```python
from build123d import *

# Parameters (mm, degrees)
SKETCH_1_W                = 290
SKETCH_1_H                = 290
EXTRUDE_1_DEPTH           = 4
EXTRUDE_2_DEPTH           = 76
SKETCH_4_W                = 6
SKETCH_4_H                = 290
EXTRUDE_3_DEPTH           = 76
CUT_EXTRUDE_12_DEPTH      = 334.95358959
CUT_EXTRUDE_12_DEPTH_BACK = 334.95358959
SKETCH_17_R               = 19.5
SKETCH_17_R_2             = 3
SKETCH_18_W               = 4
SKETCH_18_H               = 290
EXTRUDE_4_DEPTH           = 70
CUT_EXTRUDE_13_DEPTH      = 334.95358959
CUT_EXTRUDE_13_DEPTH_BACK = 334.95358959
SKETCH_14_W               = 80
SKETCH_14_H               = 30
CUT_EXTRUDE_9_DEPTH       = 20
EXTRUDE_1_2_OUTLINE_W     = 176
EXTRUDE_1_2_OUTLINE_H     = 4
EXTRUDE_1_2_DEPTH         = 20
CUT_EXTRUDE_10_DEPTH      = 334.95358959
CUT_EXTRUDE_10_DEPTH_BACK = 334.95358959
SKETCH_15_R               = 3
SKETCH_15_R_2             = 3.5
SKETCH_7_R                = 1.9
CUT_EXTRUDE_3_DEPTH       = 10
FILLET_1_R                = 2
SKETCH_21_R               = 3.6
SKETCH_21_W               = 19.5
SKETCH_21_H               = 13.5
CUT_EXTRUDE_14_DEPTH      = 10
CHAMFER_1_SIZE            = 2
FILLET_2_R                = 3
CHAMFER_2_SIZE            = 3


# Read off the part's stored shape, not the designer's step: Вытянуть-Тонкостенный1
with BuildPart() as part:
    # Эскиз1 → Extrude 1 (new body)
    with BuildSketch(Plane(origin=(0, 0, 0), x_dir=(1, 0, 0), z_dir=(0, 1, 0))):
        Rectangle(SKETCH_1_W, SKETCH_1_H)
    extrude(amount=EXTRUDE_1_DEPTH)

    # Эскиз2 → Бобышка-Вытянуть2 (add)
    with BuildSketch(Plane(origin=(0, 4, 0), x_dir=(1, 0, 0), z_dir=(0, 1, 0))):
        Polygon((145, 145), (145, 0.239524614), (145, -145), (-139, -145), (-139, -139), (139, -139), (139, 139), (-139, 139), (-139, 145), align=None)
    extrude(amount=EXTRUDE_2_DEPTH)

    # Эскиз4 → Бобышка-Вытянуть3 (add)
    with BuildSketch(Plane(origin=(0, 4, 0), x_dir=(1, 0, 0), z_dir=(0, 1, 0))):
        with Locations((-142, 0)):
            Rectangle(SKETCH_4_W, SKETCH_4_H)
    extrude(amount=EXTRUDE_3_DEPTH)

    # Эскиз17 → Вырез-Вытянуть12 (cut, two sides: drawn at the far end of the back side and taken through both)
    with BuildSketch(Plane.XY.offset(145).offset(-CUT_EXTRUDE_12_DEPTH_BACK)):
        with Locations((81, 33)):
            Circle(SKETCH_17_R)
        with Locations((57.43, 56.57)):
            Circle(SKETCH_17_R_2)
        with Locations((104.57, 56.57)):
            Circle(SKETCH_17_R_2)
        with Locations((104.57, 9.43)):
            Circle(SKETCH_17_R_2)
        with Locations((57.43, 9.43)):
            Circle(SKETCH_17_R_2)
    extrude(amount=CUT_EXTRUDE_12_DEPTH + CUT_EXTRUDE_12_DEPTH_BACK, mode=Mode.SUBTRACT)

    # Эскиз18 → Бобышка-Вытянуть4 (add)
    with BuildSketch(Plane(origin=(0, 4, 0), x_dir=(1, 0, 0), z_dir=(0, 1, 0))):
        with Locations((39, 0)):
            Rectangle(SKETCH_18_W, SKETCH_18_H)
    extrude(amount=EXTRUDE_4_DEPTH)

    # Эскиз19 → Вырез-Вытянуть13 (cut, two sides: drawn at the far end of the back side and taken through both)
    with BuildSketch(Plane(origin=(145, 0, 0), x_dir=(0, 0, -1), z_dir=(1, 0, 0)).offset(-CUT_EXTRUDE_13_DEPTH_BACK)):
        Polygon((-80, 24), (80, 24), (119, 80), (-119, 80), align=None)
    extrude(amount=CUT_EXTRUDE_13_DEPTH + CUT_EXTRUDE_13_DEPTH_BACK, mode=Mode.SUBTRACT)

    # Эскиз14 → Вырез-Вытянуть9 (cut)
    with BuildSketch(Plane(origin=(0, 4, 0), x_dir=(1, 0, 0), z_dir=(0, 1, 0))):
        with Locations((81, 120)):
            Rectangle(SKETCH_14_W, SKETCH_14_H)
        with Locations((81, -120)):
            Rectangle(SKETCH_14_W, SKETCH_14_H)
    extrude(amount=-CUT_EXTRUDE_9_DEPTH, mode=Mode.SUBTRACT)

    # Extrude 1 2 outline → Extrude 1 2 (add)
    with BuildSketch(Plane(origin=(0, 4, 0), x_dir=(1, 0, 0), z_dir=(0, 1, 0))):
        with Locations((-51, 67)):
            Rectangle(EXTRUDE_1_2_OUTLINE_W, EXTRUDE_1_2_OUTLINE_H)
        with Locations((-51, -67)):
            Rectangle(EXTRUDE_1_2_OUTLINE_W, EXTRUDE_1_2_OUTLINE_H)
    extrude(amount=EXTRUDE_1_2_DEPTH)

    # Эскиз15 → Вырез-Вытянуть10 (cut, two sides: drawn at the far end of the back side and taken through both)
    with BuildSketch(Plane.ZY.offset(145).offset(-CUT_EXTRUDE_10_DEPTH_BACK)):
        with Locations((0, 65)):
            Circle(SKETCH_15_R)
        with Locations((125, 65)):
            Circle(SKETCH_15_R_2)
        with Locations((-125, 65)):
            Circle(SKETCH_15_R_2)
        with Locations((-125, 15)):
            Circle(SKETCH_15_R_2)
        with Locations((125, 15)):
            Circle(SKETCH_15_R_2)
        with Locations((0, 15)):
            Circle(SKETCH_15_R)
    extrude(amount=CUT_EXTRUDE_10_DEPTH + CUT_EXTRUDE_10_DEPTH_BACK, mode=Mode.SUBTRACT)

    # Эскиз7 → Вырез-Вытянуть3 (cut)
    with BuildSketch(Plane(origin=(0, 4, 0), x_dir=(1, 0, 0), z_dir=(0, 1, 0))):
        with Locations(Location((-109, 55, 0), (0, 0, 270))):
            Circle(SKETCH_7_R)
        with Locations(Location((1, 55, 0), (0, 0, 90))):
            Circle(SKETCH_7_R)
        with Locations(Location((1, -55, 0), (0, 0, 270))):
            Circle(SKETCH_7_R)
        with Locations(Location((-109, -55, 0), (0, 0, 90))):
            Circle(SKETCH_7_R)
        with Locations(Location((-134, 60, 0), (0, 0, 270))):
            Circle(SKETCH_7_R)
        with Locations(Location((-134, -60, 0), (0, 0, 90))):
            Circle(SKETCH_7_R)
        with Locations(Location((134, 134, 0), (0, 0, 270))):
            Circle(SKETCH_7_R)
        with Locations(Location((134, -134, 0), (0, 0, 90))):
            Circle(SKETCH_7_R)
        with Locations(Location((134, -60, 0), (0, 0, 270))):
            Circle(SKETCH_7_R)
        with Locations(Location((134, 60, 0), (0, 0, 90))):
            Circle(SKETCH_7_R)
        with Locations(Location((46, -60, 0), (0, 0, 90))):
            Circle(SKETCH_7_R)
        with Locations(Location((46, 60, 0), (0, 0, 270))):
            Circle(SKETCH_7_R)
        with Locations(Location((45, 45, 0), (0, 0, 270))):
            Circle(SKETCH_7_R)
        with Locations(Location((135, 45, 0), (0, 0, 270))):
            Circle(SKETCH_7_R)
        with Locations(Location((45, -45, 0), (0, 0, 270))):
            Circle(SKETCH_7_R)
        with Locations(Location((135, -45, 0), (0, 0, 270))):
            Circle(SKETCH_7_R)
        with Locations(Location((-121, 124.5, 0), (0, 0, 270))):
            Circle(SKETCH_7_R)
        with Locations(Location((-121, 74.5, 0), (0, 0, 270))):
            Circle(SKETCH_7_R)
        with Locations(Location((19, 124.5, 0), (0, 0, 270))):
            Circle(SKETCH_7_R)
        with Locations(Location((19, 74.5, 0), (0, 0, 270))):
            Circle(SKETCH_7_R)
        with Locations(Location((19, -74.5, 0), (0, 0, 90))):
            Circle(SKETCH_7_R)
        with Locations(Location((19, -124.5, 0), (0, 0, 90))):
            Circle(SKETCH_7_R)
        with Locations(Location((-121, -74.5, 0), (0, 0, 90))):
            Circle(SKETCH_7_R)
        with Locations(Location((-121, -124.5, 0), (0, 0, 90))):
            Circle(SKETCH_7_R)
    extrude(amount=-CUT_EXTRUDE_3_DEPTH, mode=Mode.SUBTRACT)

    # Скругление1
    fillet_1_edges = [part.edges().sort_by_distance(p)[0] for p in [
        (-142, 24, -80),
        (-142, 24, 80),
        (39, 24, -80),
        (-139, 24, 0),
        (-51, 24, -65),
        (37, 24, 0),
        (-51, 24, 65),
        (142, 24, 80),
        (139, 4, 0),
        (139, 42, 139),
        (139, 42, -139),
        (-51, 4, 139),
        (37, 39, 139),
        (39, 74, 139),
        (41, 39, 139),
        (-139, 42, 139),
        (-139, 4, 104),
        (142, 24, -80),
        (121, 2, 135),
        (41, 2, 135),
        (41, 4, 137),
        (41, 2, 105),
        (41, 4, 0),
        (41, 2, -105),
        (41, 2, -135),
        (41, 4, -137),
        (41, 39, -139),
        (121, 2, 105),
        (121, 2, -105),
        (121, 2, -135),
        (-139, 4, -104),
        (-139, 42, -139),
        (39, 74, -139),
        (37, 39, -139),
        (-51, 4, -139),
        (-51, 4, 69),
        (37, 4, 104),
        (37, 4, -104),
        (-51, 4, -69),
        (-139, 4, 0),
        (-139, 14, -65),
        (-139, 14, 65),
        (37, 14, -65),
        (-51, 4, -65),
        (37, 4, 0),
        (37, 14, 65),
        (-51, 4, 65),
    ]]
    fillet(fillet_1_edges, radius=FILLET_1_R)

    # Эскиз21 → Вырез-Вытянуть14 (cut)
    with BuildSketch(Plane(origin=(0, 0, -145), x_dir=(-1, 0, 0), z_dir=(0, 0, -1))):
        with Locations((25, 60)):
            Circle(SKETCH_21_R)
        with Locations((75, 60)):
            Rectangle(SKETCH_21_W, SKETCH_21_H)
    extrude(amount=-CUT_EXTRUDE_14_DEPTH, mode=Mode.SUBTRACT)

    # Фаска1
    chamfer_1_edges = [part.edges().sort_by_distance(p)[0] for p in [
        (-21.4, 60, -145),
        (-84.75, 60, -145),
        (-75, 66.75, -145),
        (-65.25, 60, -145),
        (-75, 53.25, -145),
    ]]
    chamfer(chamfer_1_edges, length=CHAMFER_1_SIZE)

    # Скругление2
    fillet_2_edges = [part.edges().sort_by_distance(p)[0] for p in [
        (-84.75, 60, -143),
        (-75, 66.75, -143),
        (-65.25, 60, -143),
        (-75, 53.25, -143),
        (-21.4, 60, -143),
    ]]
    fillet(fillet_2_edges, radius=FILLET_2_R)

    # Фаска2
    chamfer_2_edges = [part.edges().sort_by_distance(p)[0] for p in [
        (54.43, 9.43, 145),
        (54.43, 9.43, -145),
        (101.57, 9.43, 145),
        (101.57, 9.43, -145),
        (101.57, 56.57, 145),
        (101.57, 56.57, -145),
        (54.43, 56.57, 145),
        (54.43, 56.57, -145),
    ]]
    chamfer(chamfer_2_edges, length=CHAMFER_2_SIZE)


solid = part.part
```
Model file for the job. Use its own axes, mm. A direction names the side the tool comes from. Give positions to 0.01 mm unless a question says otherwise; leave off trailing zeros. Loops run counter-clockwise (first coordinate to the right, second up) from the corner with the lowest first, then second, coordinate; pieces in that order, holes last. Notation, with made-up numbers: (-16.75, -22.75) -> (42.25, -22.75) arc R35 ccw to (42.25, 16.25) -> close; hole circle Ø6 at (36.25, -33.5). An arc over 180 degrees is marked (long way). Write each question's results on one line, items separated by ' | '.
(1) Cut at C-C on z = 10.5. List the corners of the cut face in (x, y).
Geometry results:
outline: (-145, 0) -> (145, 0) -> (145, 24) -> (139, 24) -> (139, 6) arc R2 cw to (137, 4) -> (43, 4) arc R2 cw to (41, 6) -> (41, 24) -> (39, 24) arc R2 ccw to (37, 22) -> (37, 6) arc R2 cw to (35, 4) -> (-137, 4) arc R2 cw to (-139, 6) -> (-139, 22) arc R2 ccw to (-141, 24) -> (-145, 24) -> close
(2) Tool access for faces 1 (the flat face through (37, 12, 1)), 2 (the conical face through (102.25, 7.3, 142.15)): list every direction of +Z, -Z, +X, -X, +Y, -Y with a clear straight run to the whole face (end or side of a thin tool).
Geometry results:
face 1: +Y | face 2: +Z
(3) Probe line 1 along X through (y, z) = (16, -115); line 2 along Z through (x, y) = (-65.5, 22.5); line 3 along Z through (x, y) = (32, 16). List the from-to ranges inside material, lowest first.
Geometry results:
line 1: x = -145 to -139, 37 to 41, 139 to 145 | line 2: z = -145 to -139, -69 to -65.06, 65.06 to 69, 139 to 145 | line 3: z = -145 to -139, -69 to -65, 65 to 69, 139 to 145
(4) Pull direction Y, two halves, no side cores. Call faces 3 (the flat face through (-142, 52, -99.5)), 4 (the cylindrical face through (-141.96, 66.05, 128.34)), 5 (the flat face through (37, 32, 111)): released by +Y, released by -Y, zero draft, split by the parting line, or undercut.
Geometry results:
face 3: released by +Y | face 4: undercut | face 5: zero draft
(5) Cut at B-B on x = -37. List the corners of the cut face in (y, z), and give its area (3 significant figures).
Geometry results:
outline: (0, -145) -> (80, -145) -> (80, -139) -> (6, -139) arc R2 cw to (4, -137) -> (4, -71) arc R2 cw to (6, -69) -> (24, -69) -> (24, -67) arc R2 ccw to (22, -65) -> (6, -65) arc R2 cw to (4, -63) -> (4, 63) arc R2 cw to (6, 65) -> (22, 65) arc R2 ccw to (24, 67) -> (24, 69) -> (6, 69) arc R2 cw to (4, 71) -> (4, 137) arc R2 cw to (6, 139) -> (80, 139) -> (80, 145) -> (0, 145) -> close | area: 2,240 mm²
(6) Cut at D-D on z = 95. List the corners of the cut face in (x, y), and give its area (3 significant figures).
Geometry results:
outline: (-145, 0) -> (145, 0) -> (145, 45.54) -> (139, 45.54) -> (139, 6) arc R2 cw to (137, 4) -> (43, 4) arc R2 cw to (41, 6) -> (41, 45.54) -> (37, 45.54) -> (37, 6) arc R2 cw to (35, 4) -> (-137, 4) arc R2 cw to (-139, 6) -> (-139, 45.54) -> (-145, 45.54) -> close | area: 1,830 mm²
(7) Cut at A-A on x = 81. List the corners of the cut face in (y, z), and give its area (3 significant figures).
Geometry results:
outline: (0, -145) -> (13.5, -145) -> (13.5, -139) -> (4, -139) -> (4, -135) -> (0, -135) -> close; (0, -105) -> (4, -105) -> (4, 105) -> (0, 105) -> close; (0, 135) -> (4, 135) -> (4, 139) -> (13.5, 139) -> (13.5, 145) -> (0, 145) -> close; (52.5, -145) -> (80, -145) -> (80, -139) -> (52.5, -139) -> close; (52.5, 139) -> (80, 139) -> (80, 145) -> (52.5, 145) -> close | area: 1,360 mm²
(8) Flat gauge pins, fed straight in: pin 1 Ø9.5 at (x, y) = (57.43, 9.43) entering from +Z; pin 2 Ø3 at (x, z) = (-81.5, -85) entering from +Y. Where does each tip first touch, or does it go through?
Geometry results:
pin 1: stops at z = 143.75 | pin 2: stops at y = 4
